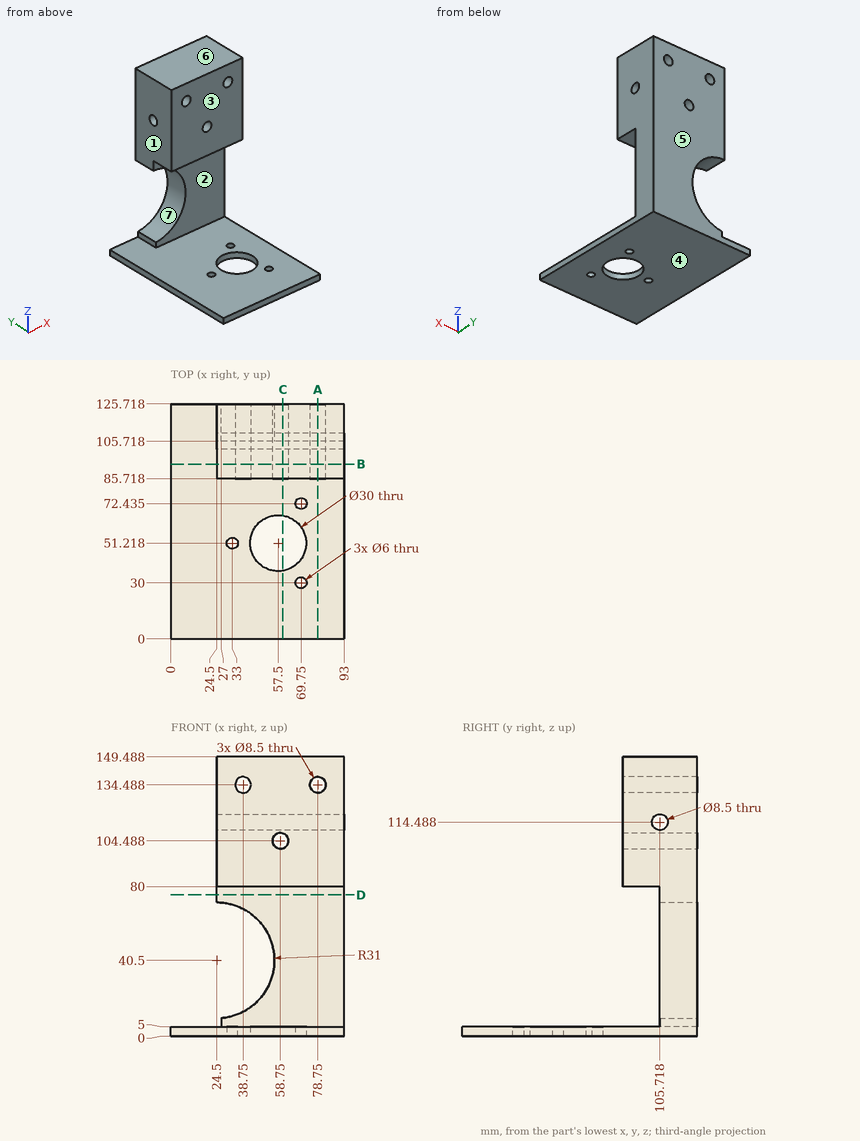
Check sheet for the drawn part. Datum: minimum x, y, z corner. Units: mm. A direction names the side the tool comes from. Give positions to 0.01 mm unless a question says otherwise; leave off trailing zeros. Write each loop counter-clockwise with the first axis right and the second up, starting at its lowest first coordinate (ties: lowest second). Pieces come first, ordered by that corner, then holes. Notation, with made-up numbers: M 46,78 L 78,78 A19 cw 78,92 Z; hole C 3.5,-22.5 d2. An arc over 180 degrees is marked long. Write item = value, one per line.
(1) Sectioned sample at A-A (x = 78.75). Record the cut outline in (y, z).
Found:
outline = M 0,0 L 125.72,0 L 125.72,130.24 L 85.72,130.24 L 85.72,80 L 105.72,80 L 105.72,5 L 0,5 Z; M 85.72,138.74 L 125.72,138.74 L 125.72,149.49 L 85.72,149.49 Z; hole C 105.72,114.49 d8.5
(2) Access from +Z, -Z, +X, -X, +Y, -Y to the whole of each face (thin tool, end or side, straight path). Record for the marked faces 1, 2, 3 and 4.
Found:
face_1 = +Z, -X, +Y, -Y
face_2 = +X, -X, -Y
face_3 = +Z, +X, -X, -Y
face_4 = -Z, +X, -X, +Y, -Y
(3) Sectioned sample at B-B (y = 93.5). Record the cut outline in (x, z).
Found:
outline = M 0,0 L 93,0 L 93,5 L 0,5 Z; M 24.5,80 L 93,80 L 93,149.49 L 24.5,149.49 Z; hole C 38.75,134.49 d8.5; hole C 58.75,104.49 d8.5; hole C 78.75,134.49 d8.5
(4) Sectioned sample at D-D (z = 75.5). Record the cut outline in (x, y), then the cut area to 3 significant figures.
Found:
outline = M 24.5,105.72 L 93,105.72 L 93,125.72 L 24.5,125.72 Z
area = 1,370 mm2
(5) Material ranges on line 1 (Z direction, x = 58.75, y = 100.5); line 2 (Y direction, x = 57.5, z = 2.1); line 3 (Z direction, x = 78.75, y = 117), recorded low to high.
Found:
line_1 = 0 to 5, 80 to 100.24, 108.74 to 149.49
line_2 = 0 to 36.22, 66.22 to 125.72
line_3 = 0 to 130.24, 138.74 to 149.49
(6) Draft check along Z on the marked faces 5, 6 and 7. Enter one of: released by +Z, released by -Z, zero draft, split by the parting line, or undercut.
Found:
face_5 = zero draft
face_6 = released by +Z
face_7 = undercut
(7) Sectioned sample at C-C (x = 60). Record the cut outline in (y, z), then the cut area to 3 significant figures.
Found:
outline = M 0,0 L 36.43,0 L 36.43,5 L 0,5 Z; M 66.01,0 L 125.72,0 L 125.72,100.43 L 85.72,100.43 L 85.72,80 L 105.72,80 L 105.72,5 L 66.01,5 Z; M 85.72,108.55 L 125.72,108.55 L 125.72,149.49 L 85.72,149.49 Z; hole C 105.72,114.49 d8.5
area = 4,380 mm2
(8) Go/stop test with flat-tipped pins: pin 1 Ø4 at (x, y) = (14, 98.5) entering from +Z; pin 2 Ø20.5 at (x, z) = (52.5, 36.5) entering from -Y; pin 3 Ø1.5 at (x, z) = (29, 120) entering from -Y; pin 4 Ø7.5 at (x, z) = (58.75, 104.488) entering from +Y. Record where each tip stops, or that it passes through.
Found:
pin_1 = 5
pin_2 = 105.72
pin_3 = 85.72
pin_4 = through
